Verification items for the finished model (mm, model axes). Face numbers are marked on the shaded views. A direction names the side the tool comes from. Round coordinates to 2 decimals unless told otherwise and drop trailing zeros. Order: outer loops, then holes, each group sorted by start corner. A loop starts at its lowest first (then second) coordinate and runs counter-clockwise, first axis right, second up. Notation, with made-up numbers: (29.5, -4.5) -> (42.5, -4.5) arc R21 cw to (42.5, 31.5) -> close; hole circle Ø6 at (20, 69). An arc over 180 degrees is marked (long way). Return JSON: item names as keys, results as strings. Group by question number.
Item 1: Depth check by flat-ended pin: pin 1 Ø4 at (x, y) = (2.5, -3) entering from +Z; pin 2 Ø1 at (y, z) = (2, 4.5) entering from +X; pin 3 Ø3 at (y, z) = (-0.5, 0.5) entering from -X. Enter the tip coordinate at first touch or a pass-through.
Item 2: Scan lines: probe 1 along Y at (x, z) = (9.5, 0); probe 2 along Z at (x, y) = (6.5, 0). Record each from-to range of solid material in increasing order. Write a range as from..to.
Item 3: Sectioned sample at D-D on x = 10. Record the cut outline in (y, z).
Item 4: Access from +Z, -Z, +X, -X, +Y, -Y to the whole of each face (thin tool, end or side, straight path). Record for the marked faces 1 and 2.
Item 5: Sectioned sample at A-A on y = 0. Record the cut outline in (x, z).
Item 6: Draft check along Y on the marked faces 3, 4 and 5. Enter one of: pulls with the +Y half, pulls with the -Y half, needs draft (parallel to the pull), parting line crosses it, or undercut.
Item 7: Sectioned sample at C-C on x = 7.25. Record the cut outline in (y, z), plus the area to 3 significant figures.
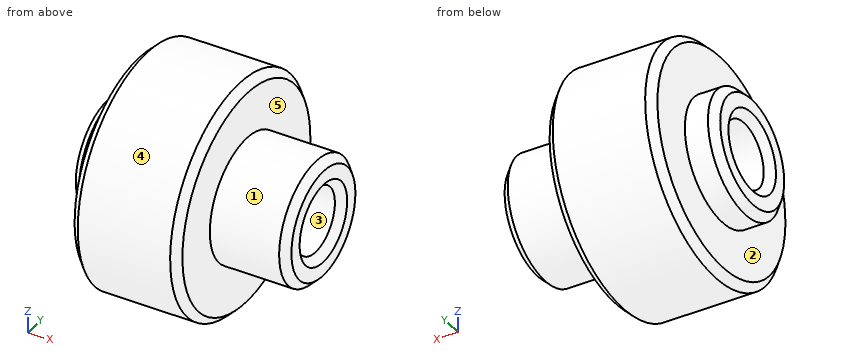
```python
from build123d import *

# Parameters (mm, degrees)
F2_SIZE = 0.5


with BuildPart() as f1:
    # F0 (on Front) → F1 (revolve)
    with BuildSketch(Plane.XZ):
        Polygon((0, 4), (0, 2.1), (14, 2.1), (14, 4), (9, 4), (9, 7.5), (2, 7.5), (2, 4), align=None)
    revolve(axis=Axis((9.418666, 0, 0), (1, 0, 0)))

    # F2
    f2_edges = [f1.edges().sort_by_distance(p)[0] for p in [
        (9, 0, -7.5),
        (2, 0, -7.5),
        (5.5, 0, 7.5),
        (0, 0, -2.1),
        (14, 0, -2.1),
        (7, 0, 2.1),
        (14, 0, -4),
        (0, 0, -4),
    ]]
    chamfer(f2_edges, length=F2_SIZE)


solid = f1.part
```
Recorded:
{
 "1": {"pin 1": "z = 7.43", "pin 2": "x = 9", "pin 3": "x = 0.39"},
 "2": {"probe 1": "-4..-2.1, 2.1..4", "probe 2": "-7.5..-2.1, 2.1..7.5"},
 "3": {"outline": "circle Ø8 at (0, 0); hole circle Ø4.2 at (0, 0)"},
 "4": {"face 1": "+X", "face 2": "-X"},
 "5": {"outline": "(0, -3.5) -> (0.5, -4) -> (2, -4) -> (2, -7) -> (2.5, -7.5) -> (8.5, -7.5) -> (9, -7) -> (9, -4) -> (13.5, -4) -> (14, -3.5) -> (14, -2.6) -> (13.5, -2.1) -> (0.5, -2.1) -> (0, -2.6) -> close; (0, 2.6) -> (0.5, 2.1) -> (13.5, 2.1) -> (14, 2.6) -> (14, 3.5) -> (13.5, 4) -> (9, 4) -> (9, 7) -> (8.5, 7.5) -> (2.5, 7.5) -> (2, 7) -> (2, 4) -> (0.5, 4) -> (0, 3.5) -> close"},
 "6": {"face 3": "undercut", "face 4": "parting line crosses it", "face 5": "needs draft"},
 "7": {"outline": "circle Ø15 at (0, 0); hole circle Ø4.2 at (0, 0)", "area": "163 mm²"}
}
